Input: part model. Units: mm. Frame: model coordinates. Give positions to 0.01 mm unless a question says otherwise; leave off trailing zeros. Write each loop counter-clockwise with the first axis right and the second up, starting at its lowest first coordinate (ties: lowest second). Pieces come first, ordered by that corner, then holes. Notation, with made-up numbers: (28, 27.25) - (65, 27.25) arc R21 ccw to (65, 55.25) - close; hole circle Ø2 at (-30, 89.25). An arc over 180 degrees is marked (long way). Use a Markdown table: item, result. Add a question column.
1. Pin query (flat end, axial travel): pin 1 (3 mm diameter, centred on y = 4, z = -36, fed in from -X). Return the tip coordinate at first contact, or that it passes through.
2. Section query B-B, the plane y = 16.25. Return loops of the section in (x, z), plus the area to 3 significant figures.
3. Material intervals for probe 1 along Y at (x, z) = (20.5, 0); probe 2 along Z at (x, y) = (-47.5, 11.25), sorted ascending.
4. Section query C-C, the plane z = 34.5. Return loops of the section in (x, y), plus the area to 3 significant figures.
5. Section query A-A, the plane x = -62. Return loops of the section in (y, z), plus the area to 3 significant figures.
```python
from build123d import *

# Parameters (mm, degrees)
SKETCH1_W           = 200
SKETCH1_H           = 210
SKETCH1_W_2         = 10
SKETCH1_H_2         = 4
SKETCH1_W_3         = 40
SKETCH1_H_3         = 15
SKETCH1_W_4         = 5
SKETCH1_H_4         = 2.5
SKETCH1_W_5         = 2.5
SKETCH1_H_5         = 5
MAINBODY_DEPTH      = 1
SKETCH1_8_W         = 40
SKETCH1_8_H         = 3.124603495
BOSS_EXTRUDE1_DEPTH = 20


with BuildPart() as part:
    # Sketch1 → MainBody (new body)
    with BuildSketch(Plane(origin=(0, 0, 0), x_dir=(1, 0, 0), z_dir=(0, 1, 0))):
        Rectangle(SKETCH1_W, SKETCH1_H)
        with Locations((89, 1)):
            Rectangle(SKETCH1_W_2, SKETCH1_H_2, mode=Mode.SUBTRACT)
        with Locations((-89, 1)):
            Rectangle(SKETCH1_W_2, SKETCH1_H_2, mode=Mode.SUBTRACT)
        with Locations((-60, 77.5)):
            Rectangle(SKETCH1_W_3, SKETCH1_H_3, mode=Mode.SUBTRACT)
        with Locations((93.5, -102.75)):
            Rectangle(SKETCH1_W_4, SKETCH1_H_4, mode=Mode.SUBTRACT)
        with Locations((0, -102.75)):
            Rectangle(SKETCH1_W_4, SKETCH1_H_4, mode=Mode.SUBTRACT)
        with Locations((-93.5, -102.75)):
            Rectangle(SKETCH1_W_4, SKETCH1_H_4, mode=Mode.SUBTRACT)
        with Locations((-83.25, 102.75)):
            Rectangle(SKETCH1_W_4, SKETCH1_H_4, mode=Mode.SUBTRACT)
        with Locations((85.75, 102.75)):
            Rectangle(SKETCH1_W_4, SKETCH1_H_4, mode=Mode.SUBTRACT)
        with Locations((97.75, -47.5)):
            Rectangle(SKETCH1_W_5, SKETCH1_H_5, mode=Mode.SUBTRACT)
        with Locations((97.75, 47.5)):
            Rectangle(SKETCH1_W_5, SKETCH1_H_5, mode=Mode.SUBTRACT)
        with Locations((-97.75, -47.5)):
            Rectangle(SKETCH1_W_5, SKETCH1_H_5, mode=Mode.SUBTRACT)
        with Locations((-97.75, 47.5)):
            Rectangle(SKETCH1_W_5, SKETCH1_H_5, mode=Mode.SUBTRACT)
    extrude(amount=MAINBODY_DEPTH)

    # Sketch1_8 → Boss-Extrude1 (add)
    with BuildSketch(Plane(origin=(0, 0, 0), x_dir=(1, 0, 0), z_dir=(0, 1, 0))):
        with Locations((-60, 71.562301748)):
            Rectangle(SKETCH1_8_W, SKETCH1_8_H)
    extrude(amount=BOSS_EXTRUDE1_DEPTH)


solid = part.part
```
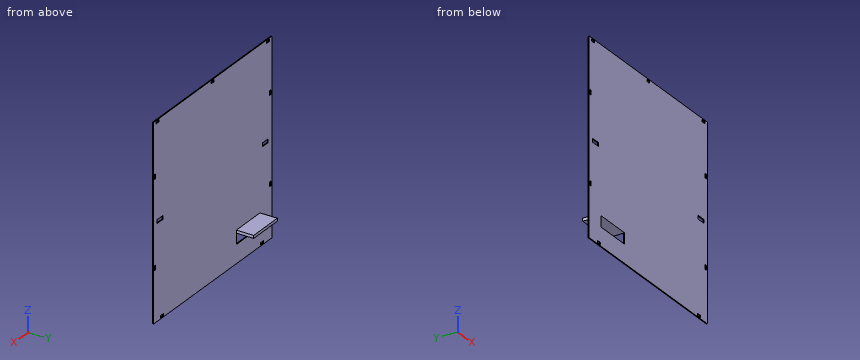
Result sheet:
| question | item | result |
|---|---|---|
| 1 | pin 1 | passes through |
| 2 | outline | (-80, -73.12) - (-40, -73.12) - (-40, -70) - (-80, -70) - close |
| 2 | area | 125 mm² |
| 3 | probe 1 | y = 0 to 1 |
| 3 | probe 2 | z = -73.12 to -70 |
| 4 | outline | (-100, 0) - (100, 0) - (100, 1) - (-100, 1) - close |
| 4 | area | 200 mm² |
| 5 | outline | (0, -105) - (1, -105) - (1, -85) - (0, -85) - close; (0, -73.12) - (20, -73.12) - (20, -70) - (1, -70) - (1, 105) - (0, 105) - close |
| 5 | area | 257 mm² |
